```python
from build123d import *

# Parameters (mm, degrees)
F0_W     = 10
F0_H     = 10
F1_DEPTH = 2
F2_W     = 10
F2_H     = 2
F3_DEPTH = 6
F4_R     = 1.5
F5_DEPTH = 25
F6_R     = 1.5
F7_DEPTH = 6
F8_W     = 1
F8_H     = 8
F9_DEPTH = 4


with BuildPart() as f1:
    # F0 (on Top) → F1 (new body)
    with BuildSketch(Plane.XY):
        Rectangle(F0_W, F0_H)
    extrude(amount=F1_DEPTH)

    # F2 (on face) → F3 (join)
    with BuildSketch(Plane.XY.offset(2)):
        with Locations((0, 4)):
            Rectangle(F2_W, F2_H)
    extrude(amount=F3_DEPTH)

    # F4 (on face) → F5 (cut)
    with BuildSketch(Plane.XZ.offset(-3)):
        with Locations((0, 5.022311)):
            Circle(F4_R)
    extrude(amount=-F5_DEPTH, mode=Mode.SUBTRACT)

    # F6 (on face) → F7 (join)
    with BuildSketch(Plane.XY.offset(2)):
        Circle(F6_R)
    extrude(amount=F7_DEPTH)

    # F8 (on face) → F9 (join)
    with BuildSketch(Plane.XY.offset(2)):
        with Locations((-4.5, -1)):
            Rectangle(F8_W, F8_H)
    extrude(amount=F9_DEPTH)


solid = f1.part
```
Read the model definition and answer for the solid it produces. Units are mm, in the model's axes. A direction names the side the tool comes from. Round coordinates to 2 decimals unless told otherwise and drop trailing zeros. Loops run counter-clockwise (first coordinate to the right, second up) from the corner with the lowest first, then second, coordinate; pieces in that order, holes last. Notation, with made-up numbers: (86.5, -25.5) -> (139.5, -25.5) arc R5 ccw to (139.5, -21.5) -> close; hole circle Ø10 at (16, 71.5). An arc over 180 degrees is marked (long way). One line per item, written item: value.
1) Consider L1, parallel to Z at x = 0, y = 4.4; L2, parallel to X at y = -2.75, z = 3.5; L3, parallel to Z at x = 1.5, y = -1.25. Determine where each line is inside the solid, lowest interval first. Write a range as [from, to].
Answer list:
L1: z = [0, 3.52], [6.52, 8]
L2: x = [-5, -4]
L3: z = [0, 2]
2) A cutting plane is placed at C-C (y = 0). Determine the outline of the cut face in (x, z).
Answer list:
outline: (-5, 0) -> (5, 0) -> (5, 2) -> (1.5, 2) -> (1.5, 8) -> (-1.5, 8) -> (-1.5, 2) -> (-4, 2) -> (-4, 6) -> (-5, 6) -> close
3) A cutting plane is placed at A-A (x = 0). Determine the outline of the cut face in (y, z), and give its area (3 significant figures).
Answer list:
outline: (-5, 0) -> (5, 0) -> (5, 3.52) -> (3, 3.52) -> (3, 2) -> (1.5, 2) -> (1.5, 8) -> (-1.5, 8) -> (-1.5, 2) -> (-5, 2) -> close; (3, 6.52) -> (5, 6.52) -> (5, 8) -> (3, 8) -> close
area: 44.0 mm²
4) For faces 1 (the face through (-4.5, -0.9, 6)), 2 (the face through (-1.5, 0.07, 4.96)), 3 (the face through (1, 3, 3.6)), 4 (the face through (0.806, 3.986, 6.287)), 5 (the face through (-4, -1, 4)), determine the directions among +Z, -Z, +X, -X, +Y, -Y from which every point of the face is accessible in a straight line to the end or side of a thin tool.
Answer list:
face 1: +Z, -X, -Y
face 2: +Z
face 3: +Z, +X
face 4: +Y
face 5: +Z, -Y
5) Flat-ended cylindrical pins translate along their axes: P1, Ø1.8, axis at x = -0.5, z = 6.5, coming from the -Y side; P2, Ø3.5, axis at x = 0, z = 5.02, coming from the +Y side; P3, Ø2, axis at y = 0, z = 4.5, coming from the +X side; P4, Ø0.5, axis at x = -4.5, y = -1.5, coming from the +Z side. Find the tip coordinate at first contact, or state that the pin passes through.
Answer list:
P1: stops at y = -1.5
P2: stops at y = 5
P3: stops at x = 1.5
P4: stops at z = 6
6) A cutting plane is placed at B-B (y = 4.5). Determine the outline of the cut face in (x, z).
Answer list:
outline: (-5, 0) -> (5, 0) -> (5, 8) -> (-5, 8) -> close; hole circle Ø3 at (0, 5.02)
7) The mould has two halves that part along X. Classify faces 6 (the face through (-5, 0, 3)), 7 (the face through (5, 2, 1)), 8 (the face through (0, -2, 2)), 9 (the face through (-1.2, -5, 1.6)): pulls with the +X half, pulls with the -X half, needs draft (parallel to the pull), parting line crosses it, or undercut.
Answer list:
face 6: pulls with the -X half
face 7: pulls with the +X half
face 8: undercut
face 9: needs draft
8) A cutting plane is placed at D-D (x = 3.75). Determine the outline of the cut face in (y, z).
Answer list:
outline: (-5, 0) -> (5, 0) -> (5, 8) -> (3, 8) -> (3, 2) -> (-5, 2) -> close
